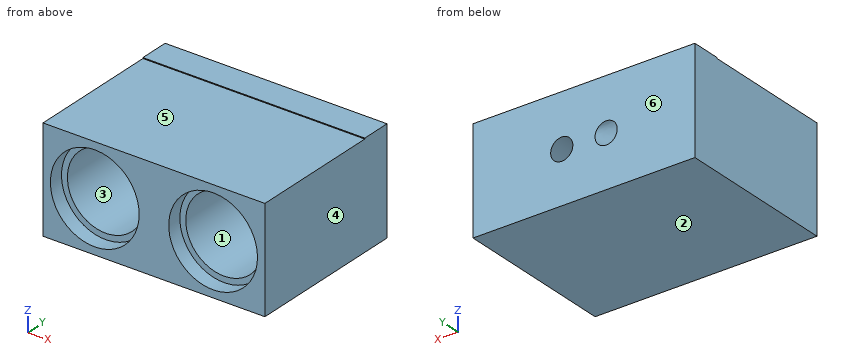
from build123d import *

# Parameters (mm, degrees)
CROQUIS1_W              = 15
CROQUIS1_H              = 7
CROQUIS1_R              = 2.6
SALIENTE_EXTRUIR1_DEPTH = 9
CROQUIS2_R              = 3
CORTAR_EXTRUIR1_DEPTH   = 1
CROQUIS3_W              = 15
CROQUIS3_H              = 7.058739116
SALIENTE_EXTRUIR2_DEPTH = 2
CROQUIS4_R              = 0.75
CROQUIS9_R              = 0.75


with BuildPart() as part:
    # Croquis1 → Saliente-Extruir1 (new body)
    with BuildSketch(Plane(origin=(0, 0, 0), x_dir=(1, 0, 0), z_dir=(0, 1, 0))):
        with Locations((-4, 0)):
            Rectangle(CROQUIS1_W, CROQUIS1_H)
        Circle(CROQUIS1_R, mode=Mode.SUBTRACT)
        with Locations((-8, 0)):
            Circle(CROQUIS1_R, mode=Mode.SUBTRACT)
    extrude(amount=SALIENTE_EXTRUIR1_DEPTH)

    # Croquis2 → Cortar-Extruir1 (cut)
    with BuildSketch(Plane.XZ):
        Circle(CROQUIS2_R)
        with Locations((-8, 0)):
            Circle(CROQUIS2_R)
    extrude(amount=-CORTAR_EXTRUIR1_DEPTH, mode=Mode.SUBTRACT)

    # Croquis3 → Saliente-Extruir2 (add)
    with BuildSketch(Plane(origin=(0, 9, 0), x_dir=(1, 0, 0), z_dir=(0, 1, 0))):
        with Locations((-4, -0.029369558)):
            Rectangle(CROQUIS3_W, CROQUIS3_H)
    extrude(amount=SALIENTE_EXTRUIR2_DEPTH)

    # Croquis4 → section 0 of cortar_recubrir3
    with BuildSketch(Plane(origin=(0, 11, 0), x_dir=(1, 0, 0), z_dir=(0, 1, 0)), mode=Mode.PRIVATE) as cortar_recubrir3_s0:
        with Locations((-5.5, -0.007482418)):
            Circle(CROQUIS4_R)
    # loft up to a face of the part (cortar_recubrir3)
    loft([cortar_recubrir3_s0.sketch, part.faces().sort_by_distance((-8, 9, 0))[0]], mode=Mode.SUBTRACT)

    # Croquis9 → section 0 of cortar_recubrir4
    with BuildSketch(Plane(origin=(0, 11, 0), x_dir=(1, 0, 0), z_dir=(0, 1, 0)), mode=Mode.PRIVATE) as cortar_recubrir4_s0:
        with Locations((-2.5, 0)):
            Circle(CROQUIS9_R)
    # loft up to a face of the part (cortar_recubrir4)
    loft([cortar_recubrir4_s0.sketch, part.faces().sort_by_distance((0, 9, 0))[0]], mode=Mode.SUBTRACT)


solid = part.part
Source: CAD feature listing. Evaluate the final solid. Frame: model axes, mm. Face numbers are marked on the shaded views. A direction names the side the tool comes from. Coordinates: 2 decimals unless noted, no trailing zeros. Loops run counter-clockwise (first coordinate to the right, second up) from the corner with the lowest first, then second, coordinate; pieces in that order, holes last. Notation, with made-up numbers: (-3.75, 60.25) -> (11.25, 60.25) arc R8 ccw to (11.25, 68.25) -> close; hole circle Ø9 at (14, -21). An arc over 180 degrees is marked (long way). Answer in a Markdown table with one row per item. Add a question column.
Q1. Reachability of the marked faces 5 and 6 from +Z, -Z, +X, -X, +Y, -Y: full face, straight path, thin tool, end or side. Return the list, or none.
Q2. Pull-direction query (Z, two-part tool) for the marked faces 1, 2, 3 and 4; classes: pulls with the +Z half, pulls with the -Z half, needs draft (parallel to the pull), parting line crosses it, or undercut.
Q3. Contact query for flat-ended pins moving along their axis: pin 1 Ø3 at (x, z) = (-7.5, 0.5) entering from -Y; pin 2 Ø5 at (x, y) = (-2.5, 2) entering from +Z. Output: stop coordinate, or through.
Q4. Ray query, line 1 along X through (y, z) = (6.25, 0); line 2 along Z through (x, y) = (0, 0.4); line 3 along X through (y, z) = (1.75, -2.25). Return the intervals inside material, ascending.
Q5. Section A-A on y = 8.5. Return the cut outline in (x, z).
Computed values:
| question | item | result |
|---|---|---|
| 1 | face 5 | +Z, +X, -X, -Y |
| 1 | face 6 | +Z, -Z, +X, -X, +Y |
| 2 | face 1 | undercut |
| 2 | face 2 | pulls with the -Z half |
| 2 | face 3 | undercut |
| 2 | face 4 | needs draft |
| 3 | pin 1 | stops at y = 9.59 |
| 3 | pin 2 | stops at z = 3.5 |
| 4 | line 1 | x = -11.5 to -10.6, -5.4 to -2.6, 2.6 to 3.5 |
| 4 | line 2 | z = -3.5 to -3, 3 to 3.5 |
| 4 | line 3 | x = -11.5 to -9.3, -6.7 to -1.3, 1.3 to 3.5 |
| 5 | outline | (-11.5, -3.5) -> (3.5, -3.5) -> (3.5, 3.5) -> (-11.5, 3.5) -> close; hole circle Ø5.2 at (-8, 0); hole circle Ø5.2 at (0, 0) |
